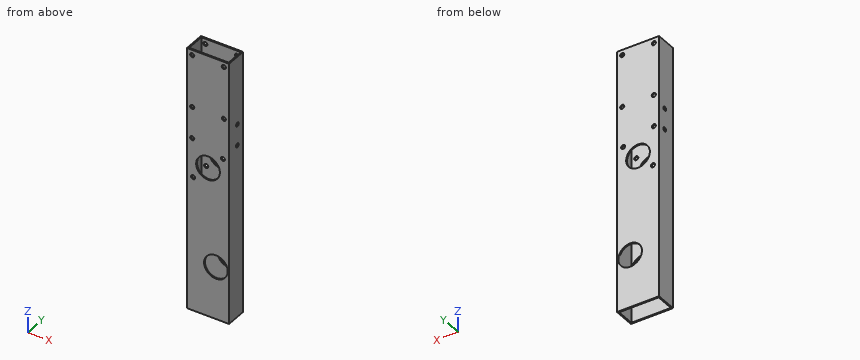
```python
from build123d import *

# Parameters (mm, degrees)
BOSS_EXTRUDE1_DEPTH      = 158.750001
BOSS_EXTRUDE1_DEPTH_BACK = 158.750001
SKETCH3_W                = 50.8
SKETCH3_H                = 25.4
SKETCH3_W_2              = 47.625
SKETCH3_H_2              = 22.225
SKETCH4_R                = 14.2875
CUT_EXTRUDE1_DEPTH       = 39.37
F_10_CLEARANCE_HOLE1_D   = 4.9784
F_10_CLEARANCE_HOLE2_D   = 4.9784
F_10_CLEARANCE_HOLE3_D   = 4.9784


with BuildPart() as part:
    # Sketch3 → Boss-Extrude1 (new, two sides: drawn at the far end of the back side and taken through both)
    with BuildSketch(Plane.XY.offset(-BOSS_EXTRUDE1_DEPTH_BACK)):
        Rectangle(SKETCH3_W, SKETCH3_H)
        Rectangle(SKETCH3_W_2, SKETCH3_H_2, mode=Mode.SUBTRACT)
    extrude(amount=BOSS_EXTRUDE1_DEPTH + BOSS_EXTRUDE1_DEPTH_BACK)

    # Sketch4 → Cut-Extrude1 (cut)
    with BuildSketch(Plane(origin=(0, 12.7, 0), x_dir=(1, 0, 0), z_dir=(0, 1, 0))):
        with Locations(Location((9.525, 95.250000508, 0), (0, 0, 180))):
            Circle(SKETCH4_R)
        with Locations(Location((0, -21.863697987, 0), (0, 0, 180))):
            Circle(SKETCH4_R)
    extrude(amount=-CUT_EXTRUDE1_DEPTH, mode=Mode.SUBTRACT)

    # #10 Clearance Hole1 (through all)
    with Locations(Plane(origin=(0, 12.7, 0), x_dir=(1, 0, 0), z_dir=(0, 1, 0))):
        with Locations((-17.960512242, -3.903185745), (17.960512242, -39.824210229)):
            Hole(F_10_CLEARANCE_HOLE1_D / 2)

    # #10 Clearance Hole2 (through all)
    with Locations(Plane.ZY.offset(25.4)):
        with Locations((50.549668409, 2.425), (75.949668409, 2.425)):
            Hole(F_10_CLEARANCE_HOLE2_D / 2)

    # #10 Clearance Hole3 (through all)
    with Locations(Plane(origin=(0, 12.7, 0), x_dir=(1, 0, 0), z_dir=(0, 1, 0))):
        with Locations((-19.05, -51.113080493), (-19.05, -89.213080493), (19.05, -89.213080493), (19.05, -152.400000508), (-19.05, -152.400000508)):
            Hole(F_10_CLEARANCE_HOLE3_D / 2)


solid = part.part
```
Verification items for the finished model (mm, model axes). Coordinates: 2 decimals unless noted, no trailing zeros. Order: outer loops, then holes, each group sorted by start corner. A loop starts at its lowest first (then second) coordinate and runs counter-clockwise, first axis right, second up. Notation, with made-up numbers: (4.5, 16.25) -> (38.5, 16.25) arc R29 ccw to (38.5, 43.25) -> close; hole circle Ø10 at (87, 46). An arc over 180 degrees is marked (long way). Put each result on its own line as item: value. Start each with the question number.
1) Material ranges on L1, parallel to X at y = -2.5, z = 38.5; L2, parallel to Y at x = -4, z = 52; L3, parallel to Z at x = 19.05, y = 12.45, recorded low to high.
2) Cross-section at B-B (y = -6.75). Enter the section's corners in (x, z), plus the area to 3 significant figures.
3) Go/stop test with a flat-tipped pin: pin 1 (10 mm diameter, centred on x = -0.5, y = 9.5, fed in from -Z). Record where the tip stops, or that it passes through.
4) Cross-section at C-C (z = -106). Enter the section's corners in (x, y).
5) Cross-section at D-D (x = 11). Enter the section's corners in (y, z), plus the area to 3 significant figures.
6) Cross-section at A-A (z = -32). Enter the section's corners in (x, y), plus the area to 3 significant figures.
Geometry check:
1. L1: x = -25.4 to -23.81, 23.81 to 25.4
1. L2: y = -12.7 to -11.11, 11.11 to 12.7
1. L3: z = -158.75 to -105.9, -84.6 to 37.59, 42.06 to 86.72, 91.7 to 149.91, 154.89 to 158.75
2. outline: (-25.4, -158.75) -> (-23.81, -158.75) -> (-23.81, 158.75) -> (-25.4, 158.75) -> close; (23.81, -158.75) -> (25.4, -158.75) -> (25.4, 158.75) -> (23.81, 158.75) -> close
2. area: 1,010 mm^2
3. pin 1: stops at z = -158.75
4. outline: (-25.4, -12.7) -> (0.11, -12.7) -> (0.11, -11.11) -> (-23.81, -11.11) -> (-23.81, 11.11) -> (0.11, 11.11) -> (0.11, 12.7) -> (-25.4, 12.7) -> close; (18.94, -12.7) -> (25.4, -12.7) -> (25.4, 12.7) -> (18.94, 12.7) -> (18.94, 11.11) -> (23.81, 11.11) -> (23.81, -11.11) -> (18.94, -11.11) -> close
5. outline: (-12.7, -158.75) -> (-11.11, -158.75) -> (-11.11, -109.46) -> (-12.7, -109.46) -> close; (-12.7, -81.04) -> (-11.11, -81.04) -> (-11.11, 12.75) -> (-12.7, 12.75) -> close; (-12.7, 30.98) -> (-11.11, 30.98) -> (-11.11, 158.75) -> (-12.7, 158.75) -> close; (11.11, -158.75) -> (12.7, -158.75) -> (12.7, -109.46) -> (11.11, -109.46) -> close; (11.11, -81.04) -> (12.7, -81.04) -> (12.7, 12.75) -> (11.11, 12.75) -> close; (11.11, 30.98) -> (12.7, 30.98) -> (12.7, 158.75) -> (11.11, 158.75) -> close
5. area: 860 mm^2
6. outline: (-25.4, -12.7) -> (25.4, -12.7) -> (25.4, 12.7) -> (-25.4, 12.7) -> close; hole (-23.81, -11.11) -> (23.81, -11.11) -> (23.81, 11.11) -> (-23.81, 11.11) -> close
6. area: 232 mm^2
